Here's how the part is built. I have some questions about the finished solid (model axes, mm). A direction names the side the tool comes from. Coordinates: 2 decimals unless noted, no trailing zeros. Loops run counter-clockwise (first coordinate to the right, second up) from the corner with the lowest first, then second, coordinate; pieces in that order, holes last. Notation, with made-up numbers: (52, -12) -> (89, -12) arc R5 ccw to (89, -5) -> close; hole circle Ø8 at (11, 69). An arc over 180 degrees is marked (long way). Answer as a JSON object with one key per item and string values. Group by question number.
1) I'm going to push a flat-ended pin straight in: pin 1 (5 mm diameter, centred on x = 97.08, y = -67.14, fed in from +Z). Where does the tip first touch, or does it pass through?
2) I need wall thicknesses on probe 1 along X at (y, z) = (4, 3.5); probe 2 along X at (y, z) = (-76, 3); probe 3 along Y at (x, z) = (95.5, 6). Which ranges of each line are inside material? Lowest first, please. Write a range as [from, to].
3) I want a section at B-B (z = 1.5). Count the separate pieces of the cut face and the enclosed holes in it, then the cut area to 3 significant figures.
4) Which directions (+Z, -Z, +X, -X, +Y, -Y) give clear straight access to the entire face, cutting with the end or side of a thin tool? Please do faces 1 (the conical face through (7.76, 50.6, 0.36)), 2 (the cylindrical face through (-26.984, -67.617, 2.247)), 3 (the conical face through (8.605, -89.381, 5.987)).
5) If we mould it in two halves opening along X, with no side actions, what happens to faces 4 (the flat face through (27.233, -19, 3)), 5 (the flat face through (13, 101.6, 3))? For each: +X half, -X half, draft (parallel to the pull), parting line (faces both ways), or undercut.
6) I want a section at A-A (y = 14.5). Write out the boundary of the cut face in (x, z).
```python
from build123d import *

# Parameters (mm, degrees)
F0_W     = 254
F0_H     = 203.2
F0_R     = 2.54
F0_R_2   = 3.175
F1_DEPTH = 6.35
F2_SIZE  = 0.508


# Not quite as in the source:
# - a fillet or chamfer that OpenCascade refuses, or shapes differently, is made with other operations: its cross-section is extruded or revolved along the edge and cut away or added


with BuildPart() as f1:
    # F0 (on Top) → F1 (new body)
    with BuildSketch(Plane.XY):
        with Locations((14.533196536, 0)):
            Rectangle(F0_W, F0_H)
        with Locations((-99.766803464, -88.9)):
            Circle(F0_R, mode=Mode.SUBTRACT)
        with Locations((-29.9168042839, -66.4009973407)):
            Circle(F0_R_2, mode=Mode.SUBTRACT)
        with Locations((-29.9168042839, -15.6009973407)):
            Circle(F0_R_2, mode=Mode.SUBTRACT)
        with BuildLine():
            ThreePointArc((27.2331968829, -70.1908171177), (8.1831968829, -89.2408171177), (-10.8668031171, -70.1908171177))
            Line((-10.8668031171, -70.1908171177), (-10.8668031171, 31.4091828823))
            ThreePointArc((-10.8668031171, 31.4091828823), (8.1831968829, 50.4591828823), (27.2331968829, 31.4091828823))
            Line((27.2331968829, 31.4091828823), (27.2331968829, -70.1908171177))
        make_face(mode=Mode.SUBTRACT)
        with Locations((128.833196536, -88.9)):
            Circle(F0_R, mode=Mode.SUBTRACT)
        with Locations((97.0831957161, -67.1428190649)):
            Circle(F0_R_2, mode=Mode.SUBTRACT)
        with Locations((97.0831957161, -16.3428190649)):
            Circle(F0_R_2, mode=Mode.SUBTRACT)
        with Locations((-99.766803464, 88.9)):
            Circle(F0_R, mode=Mode.SUBTRACT)
        with Locations((128.833196536, 88.9)):
            Circle(F0_R, mode=Mode.SUBTRACT)
    extrude(amount=F1_DEPTH)

    # F2
    f2_edges = [f1.edges().sort_by_distance(p)[0] for p in [
        (14.533197, -101.6, 6.35),
        (141.533197, 0, 6.35),
        (14.533197, 101.6, 6.35),
        (-112.466803, 0, 6.35),
        (-102.306803, -88.9, 6.35),
        (-33.091804, -66.400997, 6.35),
        (-33.091804, -15.600997, 6.35),
        (8.183197, 50.459183, 6.35),
        (27.233197, -19.390817, 6.35),
        (8.183197, -89.240817, 6.35),
        (-10.866803, -19.390817, 6.35),
        (126.293197, -88.9, 6.35),
        (93.908196, -67.142819, 6.35),
        (93.908196, -16.342819, 6.35),
        (-102.306803, 88.9, 6.35),
        (126.293197, 88.9, 6.35),
        (14.533197, -101.6, 0),
        (141.533197, 0, 0),
        (14.533197, 101.6, 0),
        (-112.466803, 0, 0),
        (-102.306803, -88.9, 0),
        (-33.091804, -66.400997, 0),
        (-33.091804, -15.600997, 0),
        (8.183197, 50.459183, 0),
        (27.233197, -19.390817, 0),
        (8.183197, -89.240817, 0),
        (-10.866803, -19.390817, 0),
        (126.293197, -88.9, 0),
        (93.908196, -67.142819, 0),
        (93.908196, -16.342819, 0),
        (-102.306803, 88.9, 0),
        (126.293197, 88.9, 0),
        (-112.466803, -101.6, 3.175),
        (-112.466803, 101.6, 3.175),
        (141.533197, -101.6, 3.175),
        (141.533197, 101.6, 3.175),
    ]]
    chamfer(f2_edges, length=F2_SIZE)

    # F3: chamfer of 5.08 on 4 edges, made by hand

    # F3_s1 → F3_t2 (revolve, cut)
    with BuildSketch(Plane.XZ.offset(66.4009973407)):
        Polygon((-21.1538042839, 6.35), (-29.8259067323, 2.7578975516), (-26.2338042839, 6.35), align=None)
    revolve(axis=Axis((-29.9168042839, -66.4009973407, 6.35), (0, 0, 1)), mode=Mode.SUBTRACT)

    # F3_s3 → F3_t4 (revolve, cut)
    with BuildSketch(Plane.XZ.offset(15.6009973407)):
        Polygon((-21.1538042839, 6.35), (-29.8259067323, 2.7578975516), (-26.2338042839, 6.35), align=None)
    revolve(axis=Axis((-29.9168042839, -15.6009973407, 6.35), (0, 0, 1)), mode=Mode.SUBTRACT)

    # F3_s5 → F3_t6 (revolve, cut)
    with BuildSketch(Plane.XZ.offset(67.1428190649)):
        Polygon((105.8461957161, 6.35), (97.1740932677, 2.7578975516), (100.7661957161, 6.35), align=None)
    revolve(axis=Axis((97.0831957161, -67.1428190649, 6.35), (0, 0, 1)), mode=Mode.SUBTRACT)

    # F3_s7 → F3_t8 (revolve, cut)
    with BuildSketch(Plane.XZ.offset(16.3428190649)):
        Polygon((105.8461957161, 6.35), (97.1740932677, 2.7578975516), (100.7661957161, 6.35), align=None)
    revolve(axis=Axis((97.0831957161, -16.3428190649, 6.35), (0, 0, 1)), mode=Mode.SUBTRACT)


solid = f1.part
```
Determined:
{
 "1": {"pin 1": "through"},
 "2": {"probe 1": "[-112.47, -10.87], [27.23, 141.53]", "probe 2": "[-112.47, -9.96], [26.33, 141.53]", "probe 3": "[-101.44, -74.9], [-59.38, -24.1], [-8.58, 101.44]"},
 "3": {"separate pieces": "1", "enclosed holes": "9", "area": "46,400 mm^2"},
 "4": {"face 1": "-Z", "face 2": "+Z, -Z", "face 3": "+Z"},
 "5": {"face 4": "undercut", "face 5": "draft"},
 "6": {"outline": "(-112.47, 0.51) -> (-111.96, 0) -> (-11.37, 0) -> (-10.87, 0.51) -> (-10.87, 5.84) -> (-11.37, 6.35) -> (-111.96, 6.35) -> (-112.47, 5.84) -> close; (27.23, 0.51) -> (27.74, 0) -> (141.03, 0) -> (141.53, 0.51) -> (141.53, 5.84) -> (141.03, 6.35) -> (27.74, 6.35) -> (27.23, 5.84) -> close"}
}
